Could you check a few things on this drawing? It's one solid part, dimensions in mm from its lowest x, y, z. A direction names the side the tool comes from. Give positions to 0.01 mm unless a question says otherwise; leave off trailing zeros. Order: outer loops, then holes, each group sorted by start corner. A loop starts at its lowest first (then second) coordinate and runs counter-clockwise, first axis right, second up. Notation, with made-up numbers: (17.5, 80.5) - (58.5, 80.5) arc R23 cw to (58.5, 107.5) - close; hole circle Ø3 at (45.25, 34). An arc over 180 degrees is marked (long way). Answer as CSV lines item,"result".
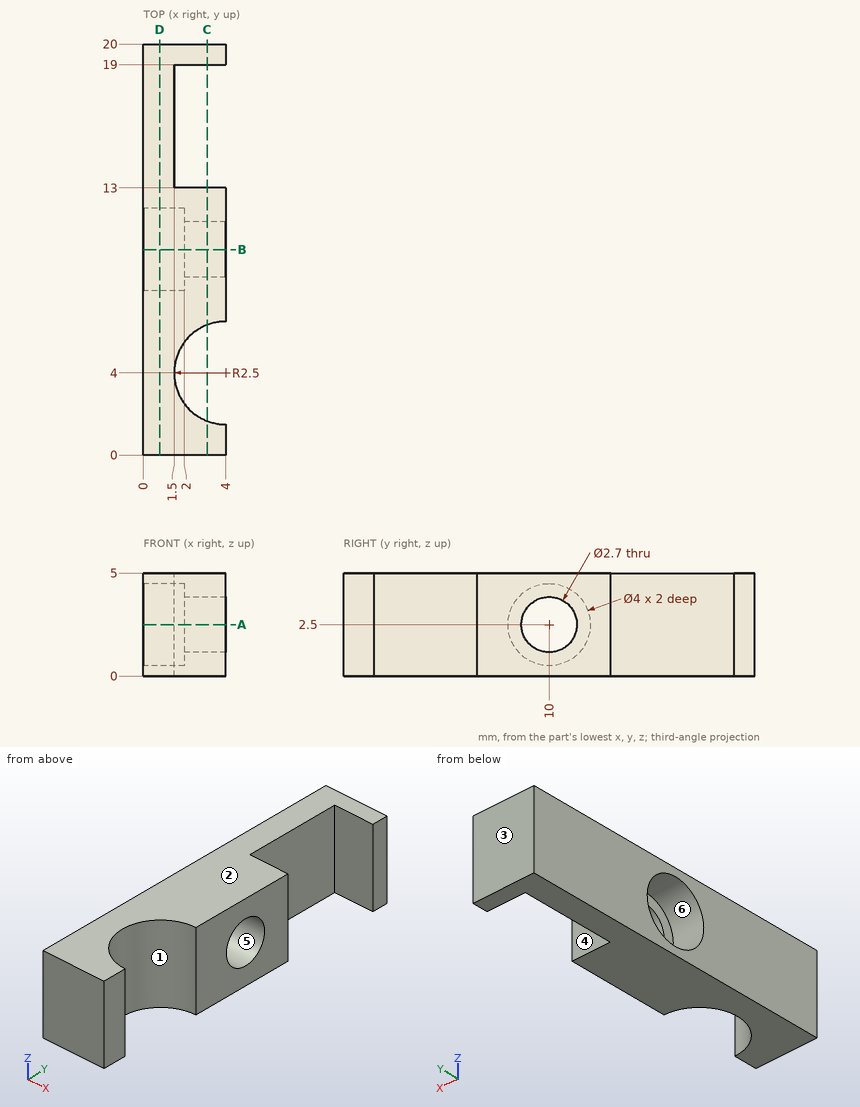
1) I want a section at D-D on x = 0.8. Write out the boundary of the cut face in (y, z), plus the area to 3 significant figures.
Answer block:
outline,"(0, 0) - (20, 0) - (20, 5) - (0, 5) - close; hole circle Ø4 at (10, 2.5)"
area,"87.4 mm2"
2) I'm going to push a flat-ended pin straight in: P1, Ø1.5, axis at y = 16.5, z = 3.5, coming from the +X side. Where does the tip first touch, or does it pass through?
Answer block:
P1,"x = 1.5"
3) I want a section at C-C on x = 3.1. Write out the boundary of the cut face in (y, z).
Answer block:
outline,"(0, 0) - (1.67, 0) - (1.67, 5) - (0, 5) - close; (6.33, 0) - (13, 0) - (13, 5) - (6.33, 5) - close; (19, 0) - (20, 0) - (20, 5) - (19, 5) - close; hole circle Ø2.7 at (10, 2.5)"
4) I want a section at B-B on y = 10. Write out the boundary of the cut face in (x, z), plus the area to 3 significant figures.
Answer block:
outline,"(0, 0) - (4, 0) - (4, 1.15) - (2, 1.15) - (2, 0.5) - (0, 0.5) - close; (0, 4.5) - (2, 4.5) - (2, 3.85) - (4, 3.85) - (4, 5) - (0, 5) - close"
area,"6.60 mm2"
5) I want a section at A-A on z = 2.5. Write out the boundary of the cut face in (x, y).
Answer block:
outline,"(0, 0) - (4, 0) - (4, 1.5) arc R2.5 cw to (4, 6.5) - (4, 8.65) - (2, 8.65) - (2, 8) - (0, 8) - close; (0, 12) - (2, 12) - (2, 11.35) - (4, 11.35) - (4, 13) - (1.5, 13) - (1.5, 19) - (4, 19) - (4, 20) - (0, 20) - close"
6) Which directions (+Z, -Z, +X, -X, +Y, -Y) give clear straight access to the entire face, cutting with the end or side of a thin tool? Please do the marked faces 4, 5 and 6.
Answer block:
face 4,"+Z, -Z, +X"
face 5,"+X, -X"
face 6,"-X"
7) If we mould it in two halves opening along Y, with no side actions, what happens to the marked faces 1, 2 and 3? For each: +Y half, -Y half, draft (parallel to the pull), parting line (faces both ways), or undercut.
Answer block:
face 1,"undercut"
face 2,"draft"
face 3,"+Y half"
8) I need wall thicknesses on line 1 along Y through (x, z) = (0.85, 2.5); line 2 along Y through (x, z) = (3.05, 2.5); line 3 along Y through (x, z) = (2.15, 2.7). Which ranges of each line are inside material? Lowest first, please. Write a range as [from, to].
Answer block:
line 1,"[0, 8], [12, 20]"
line 2,"[0, 1.69], [6.31, 8.65], [11.35, 13], [19, 20]"
line 3,"[0, 2.32], [5.68, 8.66], [11.34, 13], [19, 20]"
